```python
from build123d import *

# Parameters (mm, degrees)
F0_W     = 20
F0_H     = 20
F0_H_2   = 30
F0_W_2   = 30
F0_W_3   = 50
F0_H_3   = 50
F1_DEPTH = 20


with BuildPart() as f1:
    # F0 (on Front) → F1 (new body)
    with BuildSketch(Plane.XZ):
        with Locations((-336.827279, 390)):
            Rectangle(F0_W, F0_H)
        with Locations((-336.827279, 365)):
            Rectangle(F0_W, F0_H_2)
        with Locations((-311.827279, 390)):
            Rectangle(F0_W_2, F0_H)
        with Locations((-221.827279, 390)):
            Rectangle(F0_W_3, F0_H)
        with Locations((-121.827279, 390)):
            Rectangle(F0_W_3, F0_H)
        with Locations((-21.827279, 390)):
            Rectangle(F0_W_3, F0_H)
        with Locations((78.172721, 390)):
            Rectangle(F0_W_3, F0_H)
        with Locations((178.172721, 390)):
            Rectangle(F0_W_3, F0_H)
        with Locations((278.172721, 390)):
            Rectangle(F0_W_3, F0_H)
        with Locations((368.172721, 390)):
            Rectangle(F0_W_2, F0_H)
        with Locations((393.172721, 390)):
            Rectangle(F0_W, F0_H)
        with Locations((393.172721, 365)):
            Rectangle(F0_W, F0_H_2)
        with Locations((-336.827279, 275)):
            Rectangle(F0_W, F0_H_3)
        with Locations((-336.827279, 175)):
            Rectangle(F0_W, F0_H_3)
        with Locations((-336.827279, 75)):
            Rectangle(F0_W, F0_H_3)
        with Locations((-336.827279, -25)):
            Rectangle(F0_W, F0_H_3)
        with Locations((-336.827279, -125)):
            Rectangle(F0_W, F0_H_3)
        with Locations((-336.827279, -225)):
            Rectangle(F0_W, F0_H_3)
        with Locations((-336.827279, -315)):
            Rectangle(F0_W, F0_H_2)
        with Locations((-336.827279, -340)):
            Rectangle(F0_W, F0_H)
        with Locations((-311.827279, -340)):
            Rectangle(F0_W_2, F0_H)
        with Locations((-221.827279, -340)):
            Rectangle(F0_W_3, F0_H)
        with Locations((-121.827279, -340)):
            Rectangle(F0_W_3, F0_H)
        with Locations((-21.827279, -340)):
            Rectangle(F0_W_3, F0_H)
        with Locations((78.172721, -340)):
            Rectangle(F0_W_3, F0_H)
        with Locations((178.172721, -340)):
            Rectangle(F0_W_3, F0_H)
        with Locations((278.172721, -340)):
            Rectangle(F0_W_3, F0_H)
        with Locations((368.172721, -340)):
            Rectangle(F0_W_2, F0_H)
        with Locations((393.172721, -340)):
            Rectangle(F0_W, F0_H)
        with Locations((393.172721, -315)):
            Rectangle(F0_W, F0_H_2)
        with Locations((393.172721, -225)):
            Rectangle(F0_W, F0_H_3)
        with Locations((393.172721, -125)):
            Rectangle(F0_W, F0_H_3)
        with Locations((393.172721, -25)):
            Rectangle(F0_W, F0_H_3)
        with Locations((393.172721, 75)):
            Rectangle(F0_W, F0_H_3)
        with Locations((393.172721, 175)):
            Rectangle(F0_W, F0_H_3)
        with Locations((393.172721, 275)):
            Rectangle(F0_W, F0_H_3)
        Polygon((-296.827279, 380), (-326.827279, 380), (-326.827279, 350), (-326.827279, 300), (-326.827279, 250), (-326.827279, 200), (-326.827279, 150), (-326.827279, 100), (-326.827279, 50), (-326.827279, 0), (-326.827279, -50), (-326.827279, -100), (-326.827279, -150), (-326.827279, -200), (-326.827279, -250), (-326.827279, -300), (-326.827279, -330), (-296.827279, -330), (-246.827279, -330), (-196.827279, -330), (-146.827279, -330), (-96.827279, -330), (-46.827279, -330), (3.172721, -330), (53.172721, -330), (103.172721, -330), (153.172721, -330), (203.172721, -330), (253.172721, -330), (303.172721, -330), (353.172721, -330), (383.172721, -330), (383.172721, -300), (383.172721, -250), (383.172721, -200), (383.172721, -150), (383.172721, -100), (383.172721, -50), (383.172721, 0), (383.172721, 50), (383.172721, 100), (383.172721, 150), (383.172721, 200), (383.172721, 250), (383.172721, 300), (383.172721, 350), (383.172721, 380), (353.172721, 380), (303.172721, 380), (253.172721, 380), (203.172721, 380), (153.172721, 380), (103.172721, 380), (53.172721, 380), (3.172721, 380), (-46.827279, 380), (-96.827279, 380), (-146.827279, 380), (-196.827279, 380), (-246.827279, 380), align=None)
    extrude(amount=F1_DEPTH)


solid = f1.part
```
Geometry: final body of the model. Coordinates: model frame, mm. A direction names the side the tool comes from. Coordinates: 2 decimals unless noted, no trailing zeros. Order: outer loops, then holes, each group sorted by start corner. A loop starts at its lowest first (then second) coordinate and runs counter-clockwise, first axis right, second up. Notation, with made-up numbers: (16.5, 42.5) - (28.5, 42.5) arc R17 ccw to (28.5, 64.5) - close; hole circle Ø7 at (-0.75, -26.75). An arc over 180 degrees is marked (long way). Write each question's results on one line, items separated by ' | '.
(1) Line query: line 1 (Z direction, x = -60, y = -1); line 2 (X direction, y = -16.75, z = 303.5). Output: solid intervals per line, ascending. Write a range as [from, to].
Values found:
line 1: z = [-330, 380] | line 2: x = [-326.83, 383.17]
(2) Section query B-B, the plane x = 13.5. Return the cut outline in (y, z), plus the area to 3 significant figures.
Values found:
outline: (-20, -330) - (0, -330) - (0, 380) - (-20, 380) - close | area: 14,200 mm²
(3) Section query A-A, the plane z = 19. Return the cut outline in (x, y).
Values found:
outline: (-326.83, -20) - (383.17, -20) - (383.17, 0) - (-326.83, 0) - close
(4) First-contact query: pin 1 Ø4 at (x, y) = (252.5, -5) entering from +Z; pin 2 Ø6 at (y, z) = (-15, -59.5) entering from +X; pin 3 Ø6 at (x, y) = (119.5, -7) entering from -Z; pin 4 Ø6 at (x, y) = (331, -13.5) entering from +Z. Flat tips, straight axial feed; report the tip coordinate or a pass-through.
Values found:
pin 1: stops at z = 400 | pin 2: stops at x = 383.17 | pin 3: stops at z = -330 | pin 4: stops at z = 380
(5) Set-up query: faces 1 (the face through (229, -10, 380)), 2 (the face through (-172, -10, -330)), 3 (the face through (-337, -10, -300)), 4 (the face through (393, -10, 350)). Return all of +Z, -Z, +X, -X, +Y, -Y with unobstructed straight access to the full face (end or side cutting, diameter ignored); none if empty.
Values found:
face 1: +Z, +Y, -Y | face 2: -Z, +Y, -Y | face 3: -X, +Y, -Y | face 4: +X, +Y, -Y
(6) Mould query, pull axis Z, two halves, no side actions, for faces 5 (the face through (-337, -10, 300)), 6 (the face through (-346.827, -10, -25)), 7 (the face through (328, -10, -330)). Classes: +Z half, -Z half, draft (parallel to the pull), parting line (faces both ways), or undercut.
Values found:
face 5: undercut | face 6: draft | face 7: -Z half
